The listing builds one solid part. Answer for the finished solid, in the listing's coordinates (mm). Face numbers are marked on the shaded views. Give positions to 0.01 mm unless a question says otherwise; leave off trailing zeros. Order: outer loops, then holes, each group sorted by start corner. A loop starts at its lowest first (then second) coordinate and runs counter-clockwise, first axis right, second up. Notation, with made-up numbers: (41, -32.75) - (88, -32.75) arc R18 ccw to (88, -10.75) - close; hole circle Ø1 at (-31, -34.5). An arc over 180 degrees is marked (long way). Answer as CSV lines item,"result". Start each with the question number.
1. Section A-A on x = 0 is taken. Give the vertices of the cut face in (y, z), and give its area (3 significant figures).
2. Section B-B on y = 75 is taken. Give the vertices of the cut face in (x, z), and give its area (3 significant figures).
3. Section D-D on y = 26 is taken. Give the vertices of the cut face in (x, z).
4. Determine the mould class of the marked faces 1, 2 and 3 for opening direction X: +X half, -X half, draft (parallel to the pull), parting line (faces both ways), or undercut.
5. Flat-ended cylindrical pins translate along their axes: pin 1 (5 mm diameter, centred on x = -26, y = 99.5, fed in from +Z); pin 2 (13 mm diameter, centred on x = 0, y = 75, fed in from +Z). Find the tip coordinate at first contact, or state that the pin passes through.
6. Section C-C on z = -7 is taken. Give the vertices of the cut face in (x, y), and give its area (3 significant figures).
7. Consider line 1 along Z through (x, y) = (-27, 66.5); line 2 along Y through (x, z) = (10, -0.5); line 3 along X through (y, z) = (78.5, -7). Determine where each line is inside the solid, lowest interval first. Write a range as [from, to].
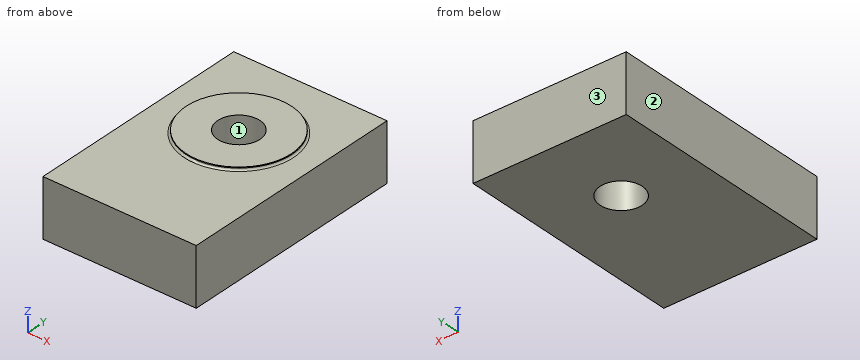
from build123d import *

# Parameters (mm, degrees)
SKETCH_1_W          = 80
SKETCH_1_H          = 30
EXTRUDE_1_DEPTH     = 120
SKETCH_2_R          = 27.5
EXTRUDE_2_DEPTH     = 1.5
SKETCH_3_R          = 11
CUT_EXTRUDE_1_DEPTH = 39.5
FILLET_1_R          = 1


with BuildPart() as part:
    # 草图1 → 凸台-拉伸1 (new body)
    with BuildSketch(Plane(origin=(0, 0, 0), x_dir=(1, 0, 0), z_dir=(0, 1, 0))):
        Rectangle(SKETCH_1_W, SKETCH_1_H)
    extrude(amount=EXTRUDE_1_DEPTH)

    # 草图2 → 凸台-拉伸2 (add)
    with BuildSketch(Plane.XY.offset(15)):
        with Locations(Location((0, 75, 0), (0, 0, 180))):
            Circle(SKETCH_2_R)
    extrude(amount=EXTRUDE_2_DEPTH)

    # 草图3 → 切除-拉伸1 (cut)
    with BuildSketch(Plane.XY.offset(16.5)):
        with Locations((0, 75)):
            Circle(SKETCH_3_R)
    extrude(amount=-CUT_EXTRUDE_1_DEPTH, mode=Mode.SUBTRACT)

    # 圆角1
    fillet_1_edges = [part.edges().sort_by_distance(p)[0] for p in [
        (27.5, 75, 15),
    ]]
    fillet(fillet_1_edges, radius=FILLET_1_R)


solid = part.part
Checks:
1,outline,"(0, -15) - (64, -15) - (64, 16.5) - (47.5, 16.5) - (47.5, 16) arc R1 cw to (46.5, 15) - (0, 15) - close; (86, -15) - (120, -15) - (120, 15) - (103.5, 15) arc R1 cw to (102.5, 16) - (102.5, 16.5) - (86, 16.5) - close"
1,area,"2,990 mm²"
2,outline,"(-40, -15) - (-11, -15) - (-11, 16.5) - (-27.5, 16.5) - (-27.5, 16) arc R1 cw to (-28.5, 15) - (-40, 15) - close; (11, -15) - (40, -15) - (40, 15) - (28.5, 15) arc R1 cw to (27.5, 16) - (27.5, 16.5) - (11, 16.5) - close"
2,area,"1,790 mm²"
3,outline,"(-40, -15) - (40, -15) - (40, 15) - (-40, 15) - close"
4,face 1,"undercut"
4,face 2,"-X half"
4,face 3,"draft"
5,pin 1,"stops at z = 15"
5,pin 2,"passes through"
6,outline,"(-40, 0) - (40, 0) - (40, 120) - (-40, 120) - close; hole circle Ø22 at (0, 75)"
6,area,"9,220 mm²"
7,line 1,"z = [-15, 15.02]"
7,line 2,"y = [0, 70.42], [79.58, 120]"
7,line 3,"x = [-40, -10.43], [10.43, 40]"
